Geometry check sheet. Reference: the model listing, model coordinates, mm. A direction names the side the tool comes from. Give positions to 0.01 mm unless a question says otherwise; leave off trailing zeros. Order: outer loops, then holes, each group sorted by start corner. A loop starts at its lowest first (then second) coordinate and runs counter-clockwise, first axis right, second up.
from build123d import *

# Parameters (mm, degrees)
CYLINDER_R        = 2.95
CYLINDER_DEPTH    = 7
CYLINDER001_R     = 1.7
CYLINDER001_DEPTH = 30


with BuildPart() as m3bolthead:
    # Cylinder → Cylinder (new body)
    with BuildSketch(Plane.XY):
        Circle(CYLINDER_R)
    extrude(amount=CYLINDER_DEPTH)


with BuildPart() as m3bolt:
    # Cylinder001 → Cylinder001 (new body)
    with BuildSketch(Plane.XY.offset(6)):
        Circle(CYLINDER001_R)
    extrude(amount=CYLINDER001_DEPTH)

    # Fusion: union M3BoltHead
    add(m3bolthead.part)


solid = m3bolt.part
Item 1: Scan lines: L1, parallel to Z at x = 2.6, y = 0.9; L2, parallel to Y at x = -1, z = 11; L3, parallel to X at y = -1.8, z = 5. Record each from-to range of solid material in increasing order.
Reported:
L1: z = 0 to 7
L2: y = -1.37 to 1.37
L3: x = -2.34 to 2.34
Item 2: Sectioned sample at A-A (y = 0). Enter the section's corners in (x, z).
Reported:
outline: (-2.95, 0) - (2.95, 0) - (2.95, 7) - (1.7, 7) - (1.7, 36) - (-1.7, 36) - (-1.7, 7) - (-2.95, 7) - close
Item 3: Sectioned sample at C-C (z = 30). Enter the section's corners in (x, y).
Reported:
outline: circle Ø3.4 at (0, 0)
Item 4: Set-up check for faces 1 (the flat face through (0, -2, 7)), 2 (the flat face through (0, 0, 0)): record each of +Z, -Z, +X, -X, +Y, -Y from which the full face is reachable in a straight line by a thin tool's end or side.
Reported:
face 1: +Z
face 2: -Z, +X, -X, +Y, -Y
Item 5: Sectioned sample at D-D (y = 2.05). Enter the section's corners in (x, z), and give its area (3 significant figures).
Reported:
outline: (-2.12, 0) - (2.12, 0) - (2.12, 7) - (-2.12, 7) - close
area: 29.7 mm2
